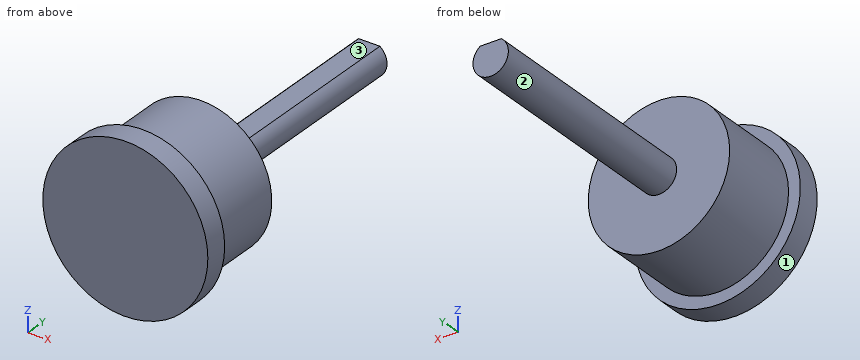
Autodesk Inventor part; units mm, degrees
ref_plane "YZ Plane" through (0, 0, 0) normal (1, 0, 0) x (0, 1, 0)
ref_plane "XZ Plane" through (0, 0, 0) normal (0, 1, 0) x (-1, 0, 0)
ref_plane "XY Plane" through (0, 0, 0) normal (0, 0, 1) x (1, 0, 0)
sketch "Sketch1" plane through (0, 0, 0) normal (0, 1, 0) x (-1, 0, 0)
  circle A0 centre (0, 0) radius 6
  dimension "d0" = 12
extrude "Extrusion1" add sketch "Sketch1" along normal blind 7
sketch "Sketch2" plane through (0, 7, 0) normal (0, 1, 0) x (1, 0, 0)
  circle A0 centre (0, 0) radius 1.5
  line L0 (-1.6953, -1.2) -> (1.8425, -1.2)
  point P0 (-0.9, -1.2)
  point P1 (0.9, -1.2)
  dimension "d3" = 3
  dimension "d5" = 2.7
extrude "Extrusion2" add sketch "Sketch2" along normal blind 20 contours A0 L0 picked at (0.3741, -0.3089)
sketch "Sketch3" plane through (0, 0, 0) normal (0, -1, 0) x (1, 0, 0)
  circle A0 centre (0, 0) radius 7
  dimension "d8" = 14
extrude "Extrusion3" add sketch "Sketch3" along normal blind 2
properties part number "spojkaRotoruSGondolou"
Check sheet for the modelled part. Datum: model origin and axes. Units: mm. Face numbers are marked on the shaded views. A direction names the side the tool comes from. Coordinates: 2 decimals unless noted, no trailing zeros. Order: outer loops, then holes, each group sorted by start corner. A loop starts at its lowest first (then second) coordinate and runs counter-clockwise, first axis right, second up. Notation, with made-up numbers: (40.25, 67) -> (54.25, 67) arc R28 ccw to (54.25, 95) -> close; hole circle Ø4 at (2, -36.75). An arc over 180 degrees is marked (long way). Write item = value, one per line. Start each with the question number.
1) Cross-section at B-B (z = 0). Enter the section's corners in (x, y), then the cut area to 3 significant figures.
2) Access from +Z, -Z, +X, -X, +Y, -Y to the whole of each face (thin tool, end or side, straight path). Record for the marked faces 1, 2 and 3.
3) Go/stop test with flat-tipped pins: P1, Ø1, axis at x = -0.5, y = 2, coming from the +Z side; P2, Ø5, axis at y = 2.5, z = 5, coming from the -X side; P3, Ø6, axis at x = 3.5, y = 14.5, coming from the -Z side. Record where each tip stops, or that it passes through.
4) Material ranges on L1, parallel to Y at x = 3.5, z = 2.25; L2, parallel to Z at x = 0, y = 9.75; L3, parallel to Y at x = 6, z = 3.5, recorded low to high.
5) Cross-section at D-D (x = -5). Enter the section's corners in (y, z), then the cut area to 3 significant figures.
6) Cross-section at A-A (x = 0). Enter the section's corners in (y, z).
7) Cross-section at C-C (y = 11.25). Enter the section's corners in (x, z).
Ans:
q1.outline = (-7, -2) -> (7, -2) -> (7, 0) -> (6, 0) -> (6, 7) -> (1.5, 7) -> (1.5, 27) -> (-1.5, 27) -> (-1.5, 7) -> (-6, 7) -> (-6, 0) -> (-7, 0) -> close
q1.area = 172 mm²
q2.face_1 = +Y, -Y
q2.face_2 = +Y
q2.face_3 = +Z, +X, -X, +Y
q3.P1 = 6
q3.P2 = -5.45
q3.P3 = -1.41
q4.L1 = -2 to 7
q4.L2 = -1.5 to 1.2
q4.L3 = -2 to 0
q5.outline = (-2, -4.9) -> (0, -4.9) -> (0, -3.32) -> (7, -3.32) -> (7, 3.32) -> (0, 3.32) -> (0, 4.9) -> (-2, 4.9) -> close
q5.area = 66.0 mm²
q6.outline = (-2, -7) -> (0, -7) -> (0, -6) -> (7, -6) -> (7, -1.5) -> (27, -1.5) -> (27, 1.2) -> (7, 1.2) -> (7, 6) -> (0, 6) -> (0, 7) -> (-2, 7) -> close
q7.outline = (-0.9, 1.2) arc R1.5 ccw (long way) to (0.9, 1.2) -> close
